from build123d import *

# Parameters (mm, degrees)
SKETCH1_W           = 67.5
SKETCH1_H           = 83
SKETCH1_W_2         = 63.5
SKETCH1_H_2         = 79
BOSS_EXTRUDE1_DEPTH = 21
SKETCH2_W           = 11
SKETCH2_H           = 17.2
SKETCH2_W_2         = 9
SKETCH2_H_2         = 15.2
BOSS_EXTRUDE2_DEPTH = 17.5
SKETCH3_W           = 9
SKETCH3_H           = 15.2
CUT_EXTRUDE1_DEPTH  = 17
FILLET1_R           = 1
SKETCH4_W           = 15
SKETCH4_H           = 6
CUT_EXTRUDE2_DEPTH  = 12


with BuildPart() as part:
    # Sketch1 → Boss-Extrude1 (new body)
    with BuildSketch(Plane.XY):
        Rectangle(SKETCH1_W, SKETCH1_H)
        Rectangle(SKETCH1_W_2, SKETCH1_H_2, mode=Mode.SUBTRACT)
    extrude(amount=BOSS_EXTRUDE1_DEPTH)

    # Sketch2 → Boss-Extrude2 (add)
    with BuildSketch(Plane(origin=(33.75, 0, 0), x_dir=(0, 0, -1), z_dir=(1, 0, 0))):
        with Locations((-11.754556837, -14.907125753)):
            Rectangle(SKETCH2_W, SKETCH2_H)
        with Locations((-11.754556837, -14.907125753)):
            Rectangle(SKETCH2_W_2, SKETCH2_H_2, mode=Mode.SUBTRACT)
    extrude(amount=BOSS_EXTRUDE2_DEPTH)

    # Sketch3 → Cut-Extrude1 (cut)
    with BuildSketch(Plane(origin=(33.75, 0, 0), x_dir=(0, 0, -1), z_dir=(1, 0, 0))):
        with Locations((-11.754556837, -14.907125753)):
            Rectangle(SKETCH3_W, SKETCH3_H)
    extrude(amount=-CUT_EXTRUDE1_DEPTH, mode=Mode.SUBTRACT)

    # Fillet1
    fillet1_edges = [part.edges().sort_by_distance(p)[0] for p in [
        (31.75, -7.307125753, 11.754556837),
    ]]
    fillet(fillet1_edges, radius=FILLET1_R)

    # Sketch4 → Cut-Extrude2 (cut)
    with BuildSketch(Plane(origin=(0, 41.5, 0), x_dir=(1, 0, 0), z_dir=(0, 1, 0))):
        with Locations((0.339523704, -8.373101697)):
            Rectangle(SKETCH4_W, SKETCH4_H)
    extrude(amount=-CUT_EXTRUDE2_DEPTH, mode=Mode.SUBTRACT)


solid = part.part
Here's how the part is built. I have some questions about the finished solid (model axes, mm). A direction names the side the tool comes from. Round coordinates to 2 decimals unless told otherwise and drop trailing zeros. Loops run counter-clockwise (first coordinate to the right, second up) from the corner with the lowest first, then second, coordinate; pieces in that order, holes last. Notation, with made-up numbers: M 27,88.25 L 79,88.25 A25 ccw 79,110.25 Z; hole C -26,38 d9. An arc over 180 degrees is marked long. Write each question's results on one line, items separated by ' | '. Start each with the question number.
(1) Thinking about a two-plate mould opening in Y: for faces 5 (the flat face through (0, 39.5, 13)), 6 (the flat face through (42, -15, 17.255)), 7 (the flat face through (31.75, -1, 10)), 8 (the flat face through (42, -23.507, 12)), which applies, pulls with the +Y half, pulls with the -Y half, needs draft (parallel to the pull), parting line crosses it, or undercut?
(2) If I drill on probe 1 along X at (y, z) = (35, 4.75); probe 2 along Y at (x, z) = (21.5, 10.25); probe 3 along X at (y, z) = (-23, 15.75), over which ranges is the centre line in solid material (lowest first)? Write a range as from..to.
(3) I want a section at C-C (y = -30). Please give me the cut outline in (x, z), then the cut area to 3 significant figures.
(4) Will these pins go through, and if not, where does the flat tip stop? P1, Ø19, axis at x = 45, y = -18, coming from the +Z side; P2, Ø9, axis at x = 46, z = 13.5, coming from the +Y side; P3, Ø4.5, axis at x = 43, z = 12, coming from the -Y side; P4, Ø12, axis at x = 1.5, y = 29.5, coming from the +Z side.
(5) On a 3-axis mill with a long thin cutter (end or side, diameter ignored), from which of +Z, -Z, +X, -X, +Y, -Y can I reach the whole of each face in a straight line? I mean faces 1 (the flat face through (-31.75, -1, 10)), 2 (the flat face through (0, 41, 11.373)), 3 (the flat face through (42, -6.307, 12)), 4 (the flat face through (42, -7.307, 12)). Say none if no direction works.
(6) I want a section at A-A (x = 13). Please give me the cut outline in (y, z), then the cut area to 3 significant figures.
(7) I want a section at D-D (x = 44.5). Please give me the cut outline in (y, z), then the cut area to 3 significant figures.
(8) I want a section at B-B (y = -12). Please give me the cut outline in (x, z), then the cut area to 3 significant figures.
Solved:
1) face 5: undercut | face 6: needs draft | face 7: undercut | face 8: pulls with the -Y half
2) probe 1: x = -33.75..-31.75, 31.75..33.75 | probe 2: y = -41.5..-39.5, 39.5..41.5 | probe 3: x = -33.75..-31.75, 31.75..51.25
3) outline: M -33.75,0 L -31.75,0 L -31.75,21 L -33.75,21 Z; M 31.75,0 L 33.75,0 L 33.75,21 L 31.75,21 Z | area: 84.0 mm²
4) P1: stops at z = 17.25 | P2: stops at y = -6.31 | P3: stops at y = -23.51 | P4: passes through
5) face 1: +Z, -Z | face 2: +Y | face 3: +Z, -Z, +X, +Y | face 4: +X
6) outline: M -41.5,0 L -39.5,0 L -39.5,21 L -41.5,21 Z; M 39.5,0 L 41.5,0 L 41.5,21 L 39.5,21 Z | area: 84.0 mm²
7) outline: M -23.51,6.25 L -6.31,6.25 L -6.31,17.25 L -23.51,17.25 Z; hole M -22.51,7.25 L -7.31,7.25 L -7.31,16.25 L -22.51,16.25 Z | area: 52.4 mm²
8) outline: M -33.75,0 L -31.75,0 L -31.75,21 L -33.75,21 Z; M 31.75,0 L 33.75,0 L 33.75,6.25 L 51.25,6.25 L 51.25,7.25 L 31.75,7.25 Z; M 31.75,16.25 L 51.25,16.25 L 51.25,17.25 L 33.75,17.25 L 33.75,21 L 31.75,21 Z | area: 101 mm²
